Geometry: see drawing. Coordinates: mm, zero at the bounding-box minimum. A direction names the side the tool comes from. Coordinates: 2 decimals unless noted, no trailing zeros. Order: outer loops, then holes, each group sorted by start corner. A loop starts at its lowest first (then second) coordinate and runs counter-clockwise, first axis right, second up.
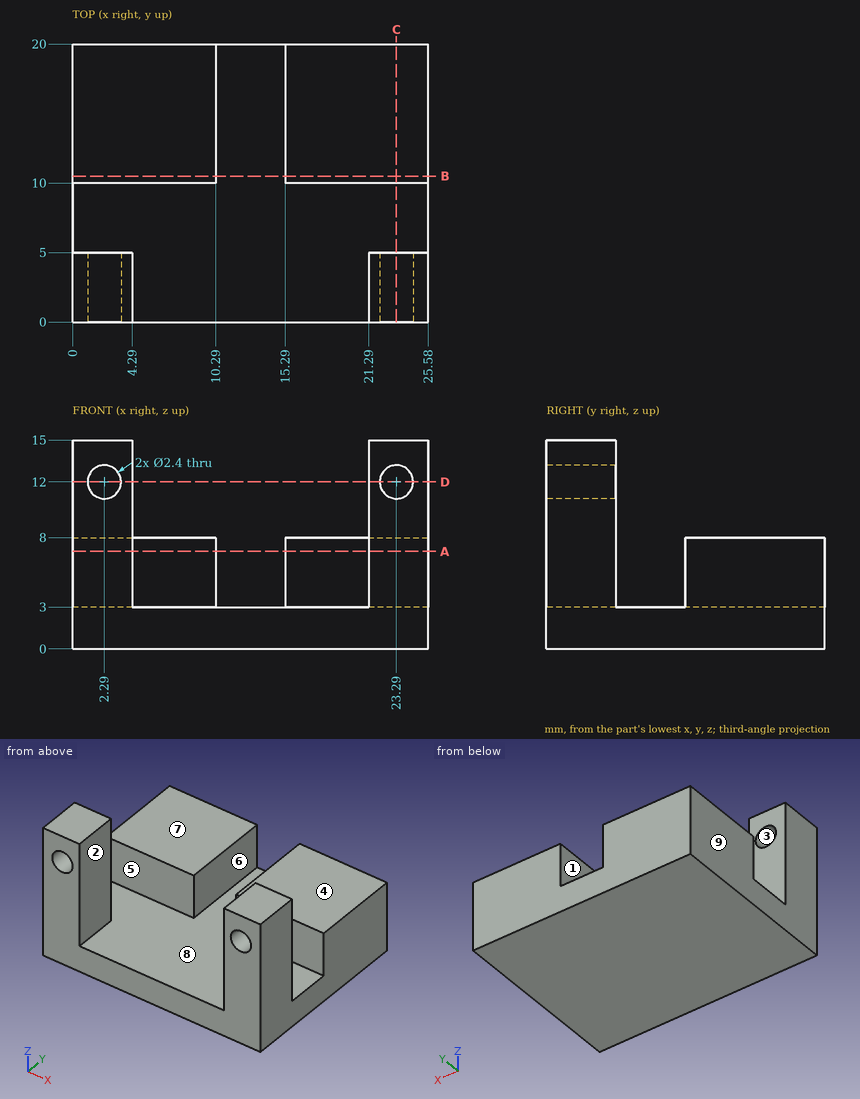
Q1. Set-up query: the marked faces 1, 2, 3, 4 and 5. Return all of +Z, -Z, +X, -X, +Y, -Y with unobstructed straight access to the full face (end or side cutting, diameter ignored); none if empty.
Solutions:
face 1: +Z, +Y, -Y
face 2: +Z, -Y
face 3: +Y, -Y
face 4: +Z, +X, -X, +Y
face 5: +Z, +X, -X
Q2. Section query D-D on z = 12. Output: boundary loops of the cut face in (x, y), plus the area to 3 significant figures.
Solutions:
outline: (0, 0) - (1.09, 0) - (1.09, 5) - (0, 5) - close; (3.49, 0) - (4.29, 0) - (4.29, 5) - (3.49, 5) - close; (21.29, 0) - (22.09, 0) - (22.09, 5) - (21.29, 5) - close; (24.49, 0) - (25.58, 0) - (25.58, 5) - (24.49, 5) - close
area: 18.9 mm2
Q3. Material intervals for line 1 along X through (y, z) = (2.05, 12); line 2 along X through (y, z) = (3.25, 4.5); line 3 along Z through (x, y) = (2.29, 3.9), sorted ascending.
Solutions:
line 1: x = 0 to 1.09, 3.49 to 4.29, 21.29 to 22.09, 24.49 to 25.58
line 2: x = 0 to 4.29, 21.29 to 25.58
line 3: z = 0 to 10.8, 13.2 to 15
Q4. Section query B-B on y = 10.5. Output: boundary loops of the cut face in (x, z), plus the area to 3 significant figures.
Solutions:
outline: (0, 0) - (25.58, 0) - (25.58, 8) - (15.29, 8) - (15.29, 3) - (10.29, 3) - (10.29, 8) - (0, 8) - close
area: 180 mm2
Q5. Pin query (flat end, axial travel): P1, Ø10, axis at x = 10.5, y = 17, coming from the -Z side; P2, Ø2.5, axis at x = 6, z = 6, coming from the -Y side; P3, Ø1.3, axis at x = 23.5, z = 9, coming from the +Y side; P4, Ø12, axis at x = 11, y = 14, coming from the +Z side. Return the tip coordinate at first contact, or that it passes through.
Solutions:
P1: stops at z = 0
P2: stops at y = 10
P3: stops at y = 5
P4: stops at z = 8
Q6. Section query C-C on x = 23.29. Output: boundary loops of the cut face in (y, z), plus the area to 3 significant figures.
Solutions:
outline: (0, 0) - (20, 0) - (20, 8) - (10, 8) - (10, 3) - (5, 3) - (5, 10.8) - (0, 10.8) - close; (0, 13.2) - (5, 13.2) - (5, 15) - (0, 15) - close
area: 158 mm2
Q7. Pull-direction query (X, two-part tool) for the marked faces 6, 7, 8 and 9; classes: pulls with the +X half, pulls with the -X half, needs draft (parallel to the pull), parting line crosses it, or undercut.
Solutions:
face 6: undercut
face 7: needs draft
face 8: undercut
face 9: pulls with the -X half
Q8. Section query A-A on z = 7. Output: boundary loops of the cut face in (x, y), plus the area to 3 significant figures.
Solutions:
outline: (0, 0) - (4.29, 0) - (4.29, 5) - (0, 5) - close; (0, 10) - (10.29, 10) - (10.29, 20) - (0, 20) - close; (15.29, 10) - (25.58, 10) - (25.58, 20) - (15.29, 20) - close; (21.29, 0) - (25.58, 0) - (25.58, 5) - (21.29, 5) - close
area: 249 mm2
